Work out the finished part from the listing and answer in its coordinate system (mm). Coordinates: 2 decimals unless noted, no trailing zeros. Order: outer loops, then holes, each group sorted by start corner. A loop starts at its lowest first (then second) coordinate and runs counter-clockwise, first axis right, second up. Notation, with made-up numbers: (50.25, 62) -> (55.25, 62) arc R12 ccw to (55.25, 73) -> close; hole circle Ø3 at (67, 46). An arc over 180 degrees is marked (long way). Write item = value, one per line. Start each with the question number.
Q1. Straight lines are drawn through the part: L1, parallel to Y at x = -16, z = -1300; L2, parallel to Y at x = 98, z = -1293.5; L3, parallel to X at y = -1410, z = -1300. For each, find the intervals that lie inside material, in ascending order. Write a range as from..to.
Q2. Flat-ended cylindrical pins translate along their axes: pin 1 (4 mm diameter, centred on y = -687.5, z = -1294, fed in from -X); pin 2 (7 mm diameter, centred on x = -53.71, z = -1300, fed in from +Y) (3 decimals). Find the tip coordinate at first contact, or state that the pin passes through.
Q3. The part is cut by section A-A, the plane y = -1352. Determine the outline of the cut face in (x, z), plus the area to 3 significant figures.
```python
from build123d import *

# Parameters (mm, degrees)
SKETCH_1_R      = 6
SKETCH_1_R_2    = 4
REVOLVE_1_ANGLE = 30
SKETCH_2_R      = 15
SKETCH_2_R_2    = 10
SKETCH_2_R_3    = 6
SKETCH_2_R_4    = 4
SKETCH_11_R     = 6
SKETCH_11_R_2   = 4
EXTRUDE_1_DEPTH = 800


with BuildPart() as part:
    # 草图1 → 旋转1 (revolve)
    with BuildSketch(Plane(origin=(0, 0, 0), x_dir=(0, 0, -1), z_dir=(1, 0, 0))):
        with Locations((1300, -0.371055822)):
            Circle(SKETCH_1_R)
        with Locations((1300, -0.371055822)):
            Circle(SKETCH_1_R_2, mode=Mode.SUBTRACT)
    revolve(axis=Axis((0, 0, -700), (0, -1, 0)), revolution_arc=REVOLVE_1_ANGLE)

    # 扫描1: sweep along a path in 草图3
    with BuildLine(Plane.YX.offset(500)) as sweep_1_path:
        Line((0, 0), (0, -21.341132523))
        ThreePointArc((0, -21.341132523), (-9.589995058, -44.493428655), (-32.742291189, -54.083423712))
        Line((-32.742291189, -54.083423712), (-932.742291189, -54.083423712))
    # 草图2 → 扫描1 (sweep)
    # profile 1 of 2: a face of its own
    with BuildSketch(Plane.ZY):
        with Locations((-500, -0.371055822)):
            Circle(SKETCH_2_R)
        with Locations((-500, -0.371055822)):
            Circle(SKETCH_2_R_2, mode=Mode.SUBTRACT)
    # profile 2 of 2: a face of its own
    with BuildSketch(Plane.ZY):
        with Locations((-1300, -0.371055822)):
            Circle(SKETCH_2_R_3)
        with Locations((-1300, -0.371055822)):
            Circle(SKETCH_2_R_4, mode=Mode.SUBTRACT)
    sweep(path=sweep_1_path.line)


with BuildPart() as sweep_1_kept_piece:
    # of the separate pieces the step leaves, the one the design keeps (sweep_1_pieces_kept)
    add(part.part.solids().sort_by_distance((0, -0.371055822, -1306))[0])

    # 草图11 → 凸台-拉伸1 (add)
    with BuildSketch(Plane.XZ.offset(932.742291189)):
        with Locations((-53.712367891, -1300)):
            Circle(SKETCH_11_R)
        with Locations((-53.712367891, -1300)):
            Circle(SKETCH_11_R_2, mode=Mode.SUBTRACT)
    extrude(amount=EXTRUDE_1_DEPTH)


solid = sweep_1_kept_piece.part
```
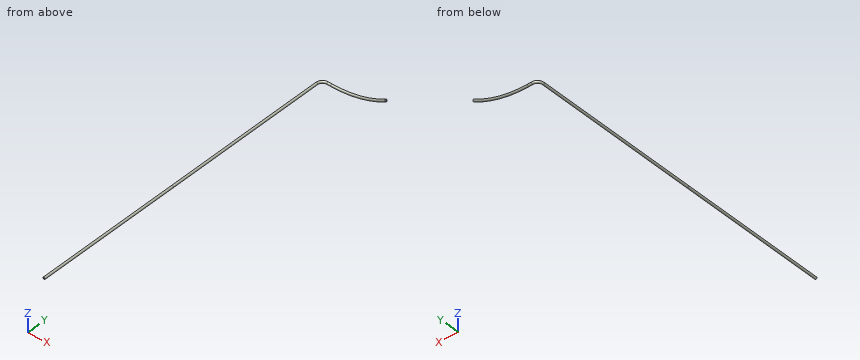
Model answer:
q1.L1 = -6.37..-4.37, 3.63..5.63
q1.L2 = -6.17..-4.06, 3.32..5.43
q1.L3 = -59.71..-57.71, -49.71..-47.71
q2.pin_1 = -58.18
q2.pin_2 = -7.465
q3.outline = circle Ø12 at (-53.71, -1300); hole circle Ø8 at (-53.71, -1300)
q3.area = 62.8 mm2
